```python
from build123d import *

# Parameters (mm, degrees)
SKETCH1_W                    = 1219.2
SKETCH1_H                    = 1016
BOSS_EXTRUDE1_DEPTH          = 3.175
F_1_4_0_25_DIAMETER_HOLE1_D  = 6.35
F_1_4_0_25_DIAMETER_HOLE2_D  = 6.35
SKETCH7_W                    = 1219.2
SKETCH7_H                    = 101.6
BOSS_EXTRUDE2_DEPTH          = 3.175
F_1_4_0_25_DIAMETER_HOLE3_D  = 6.35
FILLET1_R                    = 3.175
F_1_4_0_266_DIAMETER_HOLE1_D = 6.35


with BuildPart() as part:
    # Sketch1 → Boss-Extrude1 (new body)
    with BuildSketch(Plane.XY):
        with Locations((609.6, 508)):
            Rectangle(SKETCH1_W, SKETCH1_H)
        Polygon((1049.540905122, 508), (829.570452561, 889), (389.629547439, 889), (169.659094878, 508), (389.629547439, 127), (829.570452561, 127), align=None, mode=Mode.SUBTRACT)
    extrude(amount=BOSS_EXTRUDE1_DEPTH)

    # 1/4 (0.25) Diameter Hole1 (through all)
    with Locations(Plane.XY.offset(3.175)):
        with Locations((254, 15.875), (609.6, 15.875), (965.2, 15.875)):
            Hole(F_1_4_0_25_DIAMETER_HOLE1_D / 2)

    # 1/4 (0.25) Diameter Hole2 (through all)
    with Locations(Plane.XY.offset(3.175)):
        with Locations((1151.5725, 863.6), (67.6275, 863.6), (147.0025, 863.6), (67.6275, 152.4), (147.0025, 152.4), (67.6275, 508), (147.0025, 508), (1072.1975, 152.4), (1151.5725, 152.4), (1072.1975, 508), (1151.5725, 508), (1072.1975, 863.6)):
            Hole(F_1_4_0_25_DIAMETER_HOLE2_D / 2)

    # Sketch7 → Boss-Extrude2 (add)
    with BuildSketch(Plane.XY.offset(3.175)):
        with Locations((609.6, -50.8)):
            Rectangle(SKETCH7_W, SKETCH7_H)
    extrude(amount=-BOSS_EXTRUDE2_DEPTH)

    # 1/4 (0.25) Diameter Hole3 (through all)
    with Locations(Plane.XY.offset(3.175)):
        with Locations((965.2, -15.875), (254, -15.875), (609.6, -15.875)):
            Hole(F_1_4_0_25_DIAMETER_HOLE3_D / 2)

    # Fillet1
    fillet1_edges = [part.edges().sort_by_distance(p)[0] for p in [
        (0, -101.6, 1.5875),
        (1219.2, -101.6, 1.5875),
        (829.570452561, 127, 1.5875),
        (1049.540905122, 508, 1.5875),
        (829.570452561, 889, 1.5875),
        (389.629547439, 889, 1.5875),
        (169.659094878, 508, 1.5875),
        (389.629547439, 127, 1.5875),
        (0, 1016, 1.5875),
        (1219.2, 1016, 1.5875),
    ]]
    fillet(fillet1_edges, radius=FILLET1_R)

    # 1/4 (0.266) Diameter Hole1 (through all)
    with Locations(Plane.XY.offset(3.175)):
        with Locations((19.05, 296.333333333), (1200.15, 939.8), (1200.15, 618.066666667), (1200.15, 296.333333333), (1200.15, -25.4), (19.05, 939.8), (19.05, 618.066666667), (19.05, -25.4)):
            Hole(F_1_4_0_266_DIAMETER_HOLE1_D / 2)


solid = part.part
```
Could you check a few things on this model? Use its own coordinates, in mm. A direction names the side the tool comes from. Round coordinates to 2 decimals unless told otherwise and drop trailing zeros. Order: outer loops, then holes, each group sorted by start corner. A loop starts at its lowest first (then second) coordinate and runs counter-clockwise, first axis right, second up. Notation, with made-up numbers: M 18,-9 L 50,-9 A18 ccw 50,-2 Z; hole C 72.25,6 d3. An arc over 180 degrees is marked long. One line per question, with ' | ' between items. Start each with the question number.
(1) Suppose I cut it at B-B on y = 324. List the corners of the cut face in (x, z) for me (3 decimals).
(2) Thinking about a two-plate mould opening in X: for faces 3 (the face through (601, 92, 3.175)), 4 (the face through (938.03, 314.86, 1.57)), 5 (the face through (941, 696, 2)), which applies, +X half, -X half, draft (parallel to the pull), parting line (faces both ways), or undercut?
(3) Please list where these lines run through material, in increasing order: line 1 along X through (y, z) = (939.8, 2) (3 decimals); line 2 along Y through (x, z) = (609.6, 1.1); line 3 along Y through (x, z) = (413.5, 2.15).
(4) Suppose I cut it at A-A on x = 412.5. List the corners of the cut face in (y, z) for me (3 decimals), then the cut area to 3 significant figures.
(5) For faces 1 (the face through (601, 92, 0)), 2 (the face through (278.12, 320.14, 1.57)), which set-ups out of +Z, -Z, +X, -X, +Y, -Y let a thin tool reach every point of the face, with its end or its side?
(6) Suppose I cut it at C-C on z = 1.65. Count the separate pieces of the cut face and the enclosed holes in it, then the cut area to 3 significant figures.
Geometry results:
1) outline: M 0,0 L 275.892,0 L 275.892,3.175 L 0,3.175 Z; M 943.308,0 L 1219.2,0 L 1219.2,3.175 L 943.308,3.175 Z
2) face 3: draft | face 4: undercut | face 5: undercut
3) line 1: 0 to 15.875, 22.225 to 1196.975, 1203.325 to 1219.2 | line 2: -101.6 to -19.05, -12.7 to 12.7, 19.05 to 127, 889 to 1016 | line 3: -101.6 to 127, 889 to 1016
4) outline: M -101.6,0 L 127,0 L 127,3.175 L -101.6,3.175 Z; M 889,0 L 1016,0 L 1016,3.175 L 889,3.175 Z | area: 1,130 mm²
5) face 1: -Z, +X, -X, +Y, -Y | face 2: +Z, -Z
6) separate pieces: 1 | enclosed holes: 27 | area: 859,000 mm²
